```python
from build123d import *

# Parameters (mm, degrees)
PAD_DEPTH  = 5
SKETCH_R   = 7.5
HOLE_DEPTH = 10.001


with BuildPart() as part:
    # Sketch004 → Pad (new body, symmetric)
    with BuildSketch(Plane.XZ.offset(12.5)):
        with BuildLine():
            Line((-22.5, 59.5), (-22.5, -6e-05))
            ThreePointArc((-22.5, -6e-05), (0, -22.5), (22.5, -6e-05))
            Line((22.5, 59.5), (22.5, -6e-05))
            Line((-22.5, 59.5), (22.5, 59.5))
        make_face()
    extrude(amount=PAD_DEPTH, both=True)

    # Sketch (on Face6 of Pad) → Hole (cut, through all)
    with BuildSketch(Plane.XZ.offset(17.5)):
        Circle(SKETCH_R)
        with Locations((0, 29.5)):
            Circle(SKETCH_R)
    extrude(amount=-HOLE_DEPTH, mode=Mode.SUBTRACT)


solid = part.part
```
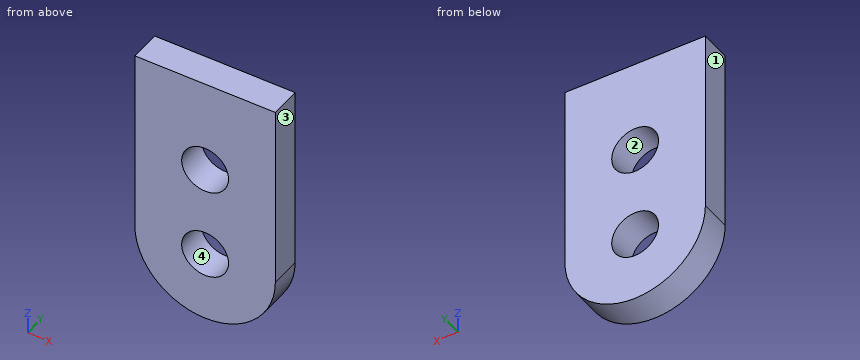
CAD build for the part. Positions are in the model's coordinates, mm. Face numbers are marked on the shaded views. Round coordinates to 2 decimals unless told otherwise and drop trailing zeros. Order: outer loops, then holes, each group sorted by start corner. A loop starts at its lowest first (then second) coordinate and runs counter-clockwise, first axis right, second up. Notation, with made-up numbers: (-2.75, 74.25) - (29.25, 74.25) arc R24 ccw to (29.25, 84.25) - close; hole circle Ø2 at (47, 8). An arc over 180 degrees is marked (long way). Answer in a Markdown table with one row per item. Add a question column.
(1) Probe L1, parallel to Z at x = 0, y = -14; L2, parallel to X at y = -13, z = 26; L3, parallel to Z at x = 9, y = -16. List the from-to ranges inside material, lowest first. Write a range as [from, to].
(2) Band-saw the part on B-B on y = -11. List the corners of the cut face in (x, z), and give its area (3 significant figures).
(3) Mould opens along X. For the marked faces 1, 2, 3 and 4 say: +X half, -X half, draft (parallel to the pull), parting line (faces both ways), or undercut.
(4) Band-saw the part on A-A on x = 0. List the corners of the cut face in (y, z).
(5) Drop a flat-ended pin along its axis: pin 1 Ø3 at (y, z) = (-14, -7) entering from -X. Give the stop position or say it passes through.
(6) Band-saw the part on D-D on z = 6.5. List the corners of the cut face in (x, y).
(7) Band-saw the part on C-C on z = 29.5. List the corners of the cut face in (x, y).
Data:
| question | item | result |
|---|---|---|
| 1 | L1 | z = [-22.5, -7.5], [7.5, 22], [37, 59.5] |
| 1 | L2 | x = [-22.5, -6.63], [6.63, 22.5] |
| 1 | L3 | z = [-20.62, 59.5] |
| 2 | outline | (-22.5, 0) arc R22.5 ccw to (22.5, 0) - (22.5, 59.5) - (-22.5, 59.5) - close; hole circle Ø15 at (0, 0); hole circle Ø15 at (0, 29.5) |
| 2 | area | 3,120 mm^2 |
| 3 | face 1 | -X half |
| 3 | face 2 | undercut |
| 3 | face 3 | +X half |
| 3 | face 4 | undercut |
| 4 | outline | (-17.5, -22.5) - (-7.5, -22.5) - (-7.5, -7.5) - (-17.5, -7.5) - close; (-17.5, 7.5) - (-7.5, 7.5) - (-7.5, 22) - (-17.5, 22) - close; (-17.5, 37) - (-7.5, 37) - (-7.5, 59.5) - (-17.5, 59.5) - close |
| 5 | pin 1 | stops at x = -21.82 |
| 6 | outline | (-22.5, -17.5) - (-3.74, -17.5) - (-3.74, -7.5) - (-22.5, -7.5) - close; (3.74, -17.5) - (22.5, -17.5) - (22.5, -7.5) - (3.74, -7.5) - close |
| 7 | outline | (-22.5, -17.5) - (-7.5, -17.5) - (-7.5, -7.5) - (-22.5, -7.5) - close; (7.5, -17.5) - (22.5, -17.5) - (22.5, -7.5) - (7.5, -7.5) - close |
